Solid Edge part; units mm, degrees
sketch "Sketch1" plane through (0, 0, 0) normal (0, 0, 1) x (1, 0, 0)
  line L0 (12.5, -13) -> (-12.5, -13)
  line L1 (-12.5, -13) -> (-12.5, 13)
  line L2 (-12.5, 13) -> (12.5, 13)
  line L3 (12.5, 13) -> (12.5, -13)
  dimension "D1" = 12.5
  dimension "D2" = 12.5
extrude "Protrusion1" add sketch "Sketch1" along normal blind 5.5
hole "Hole_1" at (-7.5, -8, 5.5) direction (0, 0, -1) diameter 2.2 end up to next
hole "Hole1" at (-7.5, 8, 5.5) direction (0, 0, -1) diameter 2.2 end up to next
hole "Hole2" at (8.5, 8, 5.5) direction (0, 0, -1) diameter 2.2 end up to next
hole "Hole3" at (8.5, -8, 5.5) direction (0, 0, -1) diameter 2.2 end up to next
sketch "Sketch2" plane through (0, 0, 0) normal (0, 0, -1) x (0, -1, 0)
  circle A0 centre (-23, -77.5) radius 25
extrude "ExtrudedProtrusion_2" add sketch "Sketch2" against normal blind 5.5
sketch "Sketch3" plane through (0, 0, 0) normal (0, 0, -1) x (-1, 0, 0)
  line L0 (-12.5, -13) -> (-81.548, -1.6701)
  line L1 (-64.5909, 44.4092) -> (-81.548, -1.6701)
  line L2 (-12.5, 13) -> (-64.5909, 44.4092)
  line L3 (-12.5, -13) -> (-12.5, 13)
extrude "ExtrudedProtrusion_5" add sketch "Sketch3" against normal blind 5.5
fillet "Round_2" radius 10 2 edges at (12.5, 13, 2.75) (12.5, -13, 2.75)
properties material "木材, アッシュ"
Work out the finished part from the listing and answer in its coordinate system (mm). A direction names the side the tool comes from. Coordinates: 2 decimals unless noted, no trailing zeros. Loops run counter-clockwise (first coordinate to the right, second up) from the corner with the lowest first, then second, coordinate; pieces in that order, holes last. Notation, with made-up numbers: (-19.5, 38.5) - (33.5, 38.5) arc R13 ccw to (33.5, 58.5) - close; hole circle Ø8 at (83, 22.25). An arc over 180 degrees is marked (long way). Use a Markdown table: item, result.
Item 1: Consider probe 1 along Y at (x, z) = (-7.5, 3.1); probe 2 along X at (y, z) = (8, 2); probe 3 along Y at (x, z) = (10, 1). Determine where each line is inside the solid, lowest interval first. Write a range as from..to.
Evaluation:
| item | result |
|---|---|
| probe 1 | y = -13..-9.1, -6.9..6.9, 9.1..13 |
| probe 2 | x = -12.5..-8.6, -6.4..7.4, 9.6..97.5 |
| probe 3 | y = -13..13 |
Item 2: Find section D-D, the plane y = 23. Determine the outline of the cut face in (x, z).
Evaluation:
| item | result |
|---|---|
| outline | (29.08, 0) - (102.5, 0) - (102.5, 5.5) - (29.08, 5.5) - close |
Item 3: For faces 1 (the cylindrical face through (8.079, 6.984, 2.788)), 2 (the flat face through (-2, 13, 3)), determine the directions among +Z, -Z, +X, -X, +Y, -Y from which every point of the face is accessible in a straight line to the end or side of a thin tool.
Evaluation:
| item | result |
|---|---|
| face 1 | +Z, -Z |
| face 2 | +Z, -Z, -X, +Y |
Item 4: The mould has two halves that part along X. Classify faces 3 (the cylindrical face through (-7.921, -9.016, 2.788)), 4 (the cylindrical face through (12.362, 13.356, 2.788)), 5 (the flat face through (46, 11, 0)): +X half, -X half, draft (parallel to the pull), parting line (faces both ways), or undercut.
Evaluation:
| item | result |
|---|---|
| face 3 | undercut |
| face 4 | -X half |
| face 5 | draft |
Item 5: Given pin 1 Ø2 at (x, z) = (23, 3.5) entering from +Y; pin 2 Ø1 at (y, z) = (40, 1.5) entering from +X; pin 3 Ø2 at (y, z) = (21, 3) entering from +X, each flat-ended and moving along its own axis, determine where each tip first touches the part or whether it passes through.
Evaluation:
| item | result |
|---|---|
| pin 1 | stops at y = 19.93 |
| pin 2 | stops at x = 96.28 |
| pin 3 | stops at x = 102.48 |
Item 6: Find section A-A, the plane y = 8. Determine the outline of the cut face in (x, z).
Evaluation:
| item | result |
|---|---|
| outline | (-12.5, 0) - (-8.6, 0) - (-8.6, 5.5) - (-12.5, 5.5) - close; (-6.4, 0) - (7.4, 0) - (7.4, 5.5) - (-6.4, 5.5) - close; (9.6, 0) - (97.5, 0) - (97.5, 5.5) - (9.6, 5.5) - close |
Item 7: Find section B-B, the plane x = 8.5. Determine the outline of the cut face in (y, z).
Evaluation:
| item | result |
|---|---|
| outline | (-13, 0) - (-9.1, 0) - (-9.1, 5.5) - (-13, 5.5) - close; (-6.9, 0) - (6.9, 0) - (6.9, 5.5) - (-6.9, 5.5) - close; (9.1, 0) - (13, 0) - (13, 5.5) - (9.1, 5.5) - close |
Item 8: Find section C-C, the plane z = 1.8. State how many separate pieces and enclosed holes the cut face has, and give its area (3 significant figures).
Evaluation:
| item | result |
|---|---|
| separate pieces | 1 |
| enclosed holes | 4 |
| area | 4,220 mm2 |
